Build history of the part. All positions in model axes, mm. A direction names the side the tool comes from. Give positions to 0.01 mm unless a question says otherwise; leave off trailing zeros. Write each loop counter-clockwise with the first axis right and the second up, starting at its lowest first coordinate (ties: lowest second). Pieces come first, ordered by that corner, then holes. Notation, with made-up numbers: (48.5, 87) -> (102.5, 87) arc R15 ccw to (102.5, 100) -> close; hole circle Ø7 at (70.25, 50). An arc over 180 degrees is marked (long way). Put each result on its own line as item: value.
from build123d import *

# Parameters (mm, degrees)
ESBO_O1_R                = 4
ESBO_O1_W                = 10
ESBO_O1_H                = 10
RESSALTO_EXTRUS_O1_DEPTH = 15


with BuildPart() as part:
    # Esboço1 → Ressalto-extrusão1 (new body)
    with BuildSketch(Plane.XY):
        with BuildLine():
            Line((78.495378078, -10.630777402), (50, 0))
            Line((50, 0), (0, 0))
            Line((0, 0), (-50, 0))
            Line((-50, 0), (-78.495378078, -10.630777402))
            ThreePointArc((-78.495378078, -10.630777402), (-84.369222598, -23.495378078), (-71.504621922, -29.369222598))
            Line((-71.504621922, -29.369222598), (-46.390791566, -20))
            Line((-46.390791566, -20), (46.390791566, -20))
            Line((46.390791566, -20), (71.504621922, -29.369222598))
            ThreePointArc((71.504621922, -29.369222598), (84.369222598, -23.495378078), (78.495378078, -10.630777402))
        make_face()
        with Locations((-50, -10)):
            Circle(ESBO_O1_R, mode=Mode.SUBTRACT)
        with Locations(Location((50, -10, 0), (0, 0, 180))):
            Circle(ESBO_O1_R, mode=Mode.SUBTRACT)
        with Locations((-75, -20)):
            Circle(ESBO_O1_R, mode=Mode.SUBTRACT)
        with Locations(Location((75, -20, 0), (0, 0, 180))):
            Circle(ESBO_O1_R, mode=Mode.SUBTRACT)
        with Locations((20, -10)):
            Rectangle(ESBO_O1_W, ESBO_O1_H, mode=Mode.SUBTRACT)
        with Locations((-20, -10)):
            Rectangle(ESBO_O1_W, ESBO_O1_H, mode=Mode.SUBTRACT)
    extrude(amount=RESSALTO_EXTRUS_O1_DEPTH)


solid = part.part
1) Pull direction Y, two halves, no side cores. Call faces 4 (the flat face through (20, -15, 7)), 5 (the cylindrical face through (84.29, -23.7, 7.4)), 6 (the cylindrical face through (-79, -20, 7)), 7 (the flat face through (1, 0, 7)): released by +Y, released by -Y, zero draft, split by the parting line, or undercut.
Filled sheet:
face 4: undercut
face 5: split by the parting line
face 6: undercut
face 7: released by +Y
2) Tool access for faces 1 (the flat face through (-1, -11, 0)), 2 (the flat face through (-1, -20, 7)), 3 (the flat face through (-15, -10, 7)): list every direction of +Z, -Z, +X, -X, +Y, -Y with a clear straight run to the whole face (end or side of a thin tool).
Filled sheet:
face 1: -Z, +X, -X, +Y, -Y
face 2: +Z, -Z, -Y
face 3: +Z, -Z
3) Slice it at C-C (x = 75). Write the cut outline in (y, z).
Filled sheet:
outline: (-30, 0) -> (-24, 0) -> (-24, 15) -> (-30, 15) -> close; (-16, 0) -> (-9.33, 0) -> (-9.33, 15) -> (-16, 15) -> close
4) Slice it at D-D (x = 9). Write the cut outline in (y, z), plus the area to 3 significant figures.
Filled sheet:
outline: (-20, 0) -> (0, 0) -> (0, 15) -> (-20, 15) -> close
area: 300 mm2
5) Pin check, flat tips, straight feed: pin 1 (3 mm diameter, centred on y = -12.5, z = 8, fed in from +X); pin 2 (1 mm diameter, centred on x = 40, z = 9, fed in from -Y); pin 3 (5 mm diameter, centred on y = -23.5, z = 9, fed in from -X); pin 4 (13 mm diameter, centred on x = 75, y = -20, fed in from +Z). Stop position of each tip, or through.
Filled sheet:
pin 1: x = 83
pin 2: y = -20
pin 3: x = -84.95
pin 4: z = 15
6) Slice it at B-B (y = -26). Write the cut outline in (x, z).
Filled sheet:
outline: (-83, 0) -> (-62.47, 0) -> (-62.47, 15) -> (-83, 15) -> close; (62.47, 0) -> (83, 0) -> (83, 15) -> (62.47, 15) -> close
7) Slice it at A-A (z = 10.25). Write the cut outline in (x, y), plus the area to 3 significant figures.
Filled sheet:
outline: (-78.5, -10.63) arc R10 ccw to (-71.5, -29.37) -> (-46.39, -20) -> (46.39, -20) -> (71.5, -29.37) arc R10 ccw to (78.5, -10.63) -> (50, 0) -> (-50, 0) -> close; hole circle Ø8 at (-75, -20); hole circle Ø8 at (-50, -10); hole (-25, -15) -> (-15, -15) -> (-15, -5) -> (-25, -5) -> close; hole (15, -15) -> (25, -15) -> (25, -5) -> (15, -5) -> close; hole circle Ø8 at (50, -10); hole circle Ø8 at (75, -20)
area: 2,990 mm2
8) Wall check: L1, parallel to X at y = -19.25, z = 5.5; L2, parallel to Y at x = 36, z = 2.75; L3, parallel to Y at x = -50, z = 9.5. Give the ranges that are in metal, low to high.
Filled sheet:
L1: -84.97 to -78.93, -71.07 to 71.07, 78.93 to 84.97
L2: -20 to 0
L3: -21.35 to -14, -6 to 0
